Autodesk Fusion 360 part; units mm, degrees
sketch "Sketch1" plane through (0, 0, 0) normal (0, 0, 1) x (1, 0, 0)
  line L0 (242.5602, 1007.653) -> (332.5602, 1007.653)
  line L1 (232.5602, 997.653) -> (232.5602, 952)
  line L2 (229.5602, 949) -> (212.5602, 949)
  line L3 (209.5602, 946) -> (209.5602, 940)
  line L4 (209.5602, 940) -> (229.5602, 940)
  arc A0 (242.5602, 1007.653) -> (232.5602, 997.653) centre (242.5602, 997.653) ccw
  line L5 (260.5602, 982.653) -> (332.5602, 982.653)
  line L6 (229.5602, 928) -> (209.5602, 928)
  line L7 (209.5602, 928) -> (209.5602, 921.1082)
  line L8 (212.5602, 918.1082) -> (227.6643, 918.1082)
  line L9 (229.5602, 940) -> (232.5602, 940)
  line L10 (229.5602, 928) -> (232.5602, 928)
  arc A1 (232.5602, 928) -> (232.5602, 940) centre (232.5602, 934) ccw
  line L11 (230.6643, 915.1082) -> (230.6643, 842.653)
  line L12 (257.5602, 979.653) -> (257.5602, 842.653)
  arc A2 (229.5602, 949) -> (232.5602, 952) centre (229.5602, 952) ccw
  arc A3 (230.6643, 915.1082) -> (227.6643, 918.1082) centre (227.6643, 915.1082) ccw
  arc A4 (212.5602, 949) -> (209.5602, 946) centre (212.5602, 946) ccw
  arc A5 (209.5602, 921.1082) -> (212.5602, 918.1082) centre (212.5602, 921.1082) ccw
  line L13 (435.5602, 949) -> (452.5602, 949)
  arc A6 (432.5602, 940) -> (432.5602, 928) centre (432.5602, 934) ccw
  line L14 (435.5602, 928) -> (432.5602, 928)
  line L15 (407.5602, 979.653) -> (407.5602, 842.653)
  line L16 (434.4561, 915.1082) -> (434.4561, 842.653)
  arc A7 (432.5602, 952) -> (435.5602, 949) centre (435.5602, 952) ccw
  line L17 (452.5602, 918.1082) -> (437.4561, 918.1082)
  arc A8 (432.5602, 997.653) -> (422.5602, 1007.653) centre (422.5602, 997.653) ccw
  line L18 (435.5602, 940) -> (432.5602, 940)
  arc A9 (437.4561, 918.1082) -> (434.4561, 915.1082) centre (437.4561, 915.1082) ccw
  arc A10 (452.5602, 918.1082) -> (455.5602, 921.1082) centre (452.5602, 921.1082) ccw
  line L19 (455.5602, 940) -> (435.5602, 940)
  line L20 (455.5602, 946) -> (455.5602, 940)
  line L21 (455.5602, 928) -> (455.5602, 921.1082)
  line L22 (422.5602, 1007.653) -> (332.5602, 1007.653)
  line L23 (404.5602, 982.653) -> (332.5602, 982.653)
  line L24 (432.5602, 997.653) -> (432.5602, 952)
  line L25 (435.5602, 928) -> (455.5602, 928)
  arc A11 (455.5602, 946) -> (452.5602, 949) centre (452.5602, 946) ccw
  line L26 (435.5602, 757.3059) -> (432.5602, 757.3059)
  line L27 (232.5602, 687.653) -> (232.5602, 733.3059)
  arc A12 (227.6643, 767.1978) -> (230.6643, 770.1978) centre (227.6643, 770.1978) ccw
  arc A13 (435.5602, 736.3059) -> (432.5602, 733.3059) centre (435.5602, 733.3059) ccw
  line L28 (212.5602, 767.1978) -> (227.6643, 767.1978)
  line L29 (455.5602, 757.3059) -> (455.5602, 764.1978)
  line L30 (229.5602, 757.3059) -> (232.5602, 757.3059)
  line L31 (435.5602, 736.3059) -> (452.5602, 736.3059)
  arc A14 (422.5602, 677.653) -> (432.5602, 687.653) centre (422.5602, 687.653) ccw
  line L32 (209.5602, 745.3059) -> (229.5602, 745.3059)
  arc A15 (209.5602, 739.3059) -> (212.5602, 736.3059) centre (212.5602, 739.3059) ccw
  arc A16 (232.5602, 733.3059) -> (229.5602, 736.3059) centre (229.5602, 733.3059) ccw
  arc A17 (232.5602, 687.653) -> (242.5602, 677.653) centre (242.5602, 687.653) ccw
  line L33 (455.5602, 739.3059) -> (455.5602, 745.3059)
  arc A18 (455.5602, 764.1978) -> (452.5602, 767.1978) centre (452.5602, 764.1978) ccw
  line L34 (209.5602, 757.3059) -> (209.5602, 764.1978)
  line L35 (229.5602, 745.3059) -> (232.5602, 745.3059)
  line L36 (209.5602, 739.3059) -> (209.5602, 745.3059)
  arc A19 (432.5602, 757.3059) -> (432.5602, 745.3059) centre (432.5602, 751.3059) ccw
  line L37 (455.5602, 745.3059) -> (435.5602, 745.3059)
  arc A20 (434.4561, 770.1978) -> (437.4561, 767.1978) centre (437.4561, 770.1978) ccw
  line L38 (435.5602, 757.3059) -> (455.5602, 757.3059)
  line L39 (432.5602, 687.653) -> (432.5602, 733.3059)
  line L40 (452.5602, 767.1978) -> (437.4561, 767.1978)
  line L41 (435.5602, 745.3059) -> (432.5602, 745.3059)
  arc A21 (452.5602, 736.3059) -> (455.5602, 739.3059) centre (452.5602, 739.3059) ccw
  arc A22 (212.5602, 767.1978) -> (209.5602, 764.1978) centre (212.5602, 764.1978) ccw
  line L42 (229.5602, 736.3059) -> (212.5602, 736.3059)
  line L43 (260.5602, 702.653) -> (332.5602, 702.653)
  line L44 (404.5602, 702.653) -> (332.5602, 702.653)
  arc A23 (232.5602, 745.3059) -> (232.5602, 757.3059) centre (232.5602, 751.3059) ccw
  line L45 (242.5602, 677.653) -> (332.5602, 677.653)
  line L46 (422.5602, 677.653) -> (332.5602, 677.653)
  line L47 (229.5602, 757.3059) -> (209.5602, 757.3059)
  line L48 (230.6643, 842.653) -> (230.6643, 770.1978)
  line L49 (257.5602, 842.653) -> (257.5602, 705.653)
  line L50 (407.5602, 842.653) -> (407.5602, 705.653)
  line L51 (434.4561, 842.653) -> (434.4561, 770.1978)
  arc A24 (407.5602, 979.653) -> (404.5602, 982.653) centre (404.5602, 979.653) ccw
  arc A25 (404.5602, 702.653) -> (407.5602, 705.653) centre (404.5602, 705.653) ccw
  arc A26 (260.5602, 982.653) -> (257.5602, 979.653) centre (260.5602, 979.653) ccw
  arc A27 (257.5602, 705.653) -> (260.5602, 702.653) centre (260.5602, 705.653) ccw
  point P0 (750, 0)
  point P1 (232.5602, 1007.653)
  point P2 (432.5602, 1007.653)
  point P3 (232.5602, 677.653)
  point P4 (432.5602, 677.653)
  dimension "d18" = 10
  dimension "d28" = 25
  dimension "d59" = 3
  dimension "d60" = 3
  dimension "d61" = 3
  dimension "d62" = 3
  dimension "d63" = 3
  dimension "d64" = 3
  dimension "d65" = 3
  dimension "d66" = 3
extrude "Extrude1" add sketch "Sketch1" along normal blind 15
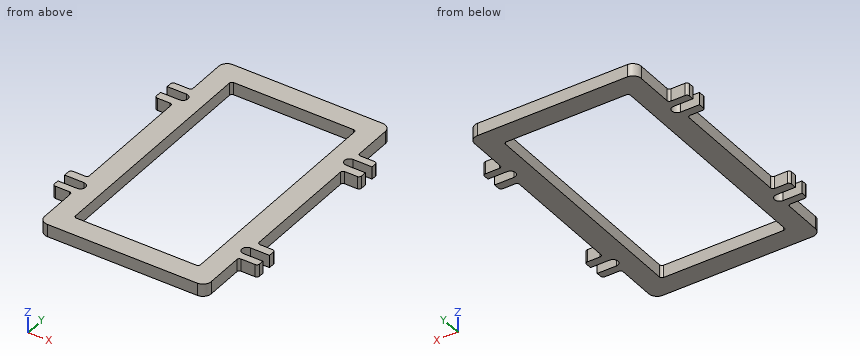
Input: part model. Units: mm. Frame: model coordinates. Coordinates: 2 decimals unless noted, no trailing zeros. Loops run counter-clockwise (first coordinate to the right, second up) from the corner with the lowest first, then second, coordinate; pieces in that order, holes last.
Q1. Cut plane A-A (x = 285). Output: boundary loops of the cut face in (y, z), then the cut area to 3 significant figures.
Q2. Contact query for flat-ended pins moving along their axis: pin 1 (7.5 mm diameter, centred on x = 440, z = 4.5, fed in from +Y); pin 2 (1 mm diameter, centred on y = 766, z = 10.5, fed in from -X); pin 3 (7.5 mm diameter, centred on x = 442.5, z = 8, fed in from -Y). Output: stop coordinate, or through.
Q3. Material intervals for line 1 (Y direction, x = 226, z = 1); line 2 (X direction, y = 967, z = 14.25); line 3 (Y direction, x = 345, z = 5.25), sorted ascending.
Q4. Cut plane B-B (y = 934). Output: boundary loops of the cut face in (x, z), then the cut area to 3 significant figures.
Working result:
1. outline: (677.65, 0) - (702.65, 0) - (702.65, 15) - (677.65, 15) - close; (982.65, 0) - (1007.65, 0) - (1007.65, 15) - (982.65, 15) - close
1. area: 750 mm2
2. pin 1: stops at y = 949
2. pin 2: stops at x = 209.86
2. pin 3: stops at y = 736.31
3. line 1: y = 736.31 to 745.31, 757.31 to 767.2, 918.11 to 928, 940 to 949
3. line 2: x = 232.56 to 257.56, 407.56 to 432.56
3. line 3: y = 677.65 to 702.65, 982.65 to 1007.65
4. outline: (238.56, 0) - (257.56, 0) - (257.56, 15) - (238.56, 15) - close; (407.56, 0) - (426.56, 0) - (426.56, 15) - (407.56, 15) - close
4. area: 570 mm2
